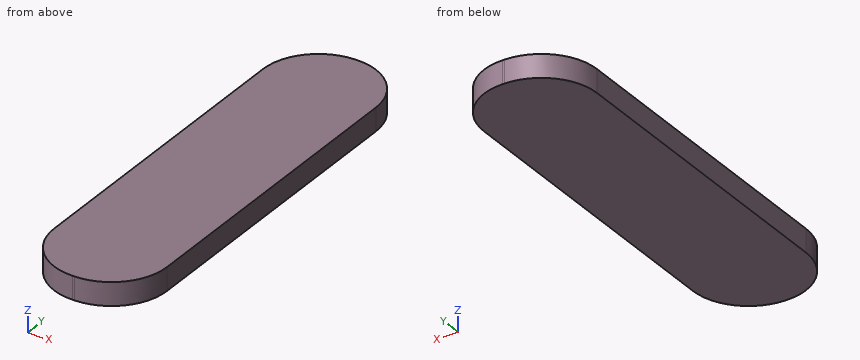
```python
from build123d import *

# Parameters (mm, degrees)
SKETCH1_W           = 12.2
SKETCH1_H           = 45.8
BOSS_EXTRUDE1_DEPTH = 2.5
FILLET1_R           = 6


with BuildPart() as part:
    # Sketch1 → Boss-Extrude1 (new body)
    with BuildSketch(Plane.XY.offset(10)):
        with Locations((-182.131179691, 159.988166791)):
            Rectangle(SKETCH1_W, SKETCH1_H)
    extrude(amount=BOSS_EXTRUDE1_DEPTH)

    # Fillet1
    fillet1_edges = [part.edges().sort_by_distance(p)[0] for p in [
        (-188.231179691, 182.888166791, 11.25),
        (-176.031179691, 182.888166791, 11.25),
        (-176.031179691, 137.088166791, 11.25),
        (-188.231179691, 137.088166791, 11.25),
    ]]
    fillet(fillet1_edges, radius=FILLET1_R)


solid = part.part
```
Geometry: final body of the model. Coordinates: model frame, mm. Coordinates: 2 decimals unless noted, no trailing zeros. Order: outer loops, then holes, each group sorted by start corner. A loop starts at its lowest first (then second) coordinate and runs counter-clockwise, first axis right, second up. Notation, with made-up numbers: M 74,58.5 L 119,58.5 A32 ccw 119,95.5 Z; hole C 84,30.5 d7. An arc over 180 degrees is marked long. Answer as CSV lines item,"result".
Q1. Section C-C on y = 142. Return the cut outline in (x, z), and give its area (3 significant figures).
Answers:
outline,"M -188.13,10 L -176.13,10 L -176.13,12.5 L -188.13,12.5 Z"
area,"30.0 mm^2"
Q2. Section A-A on z = 11.5. Return the cut outline in (x, y).
Answers:
outline,"M -188.23,143.09 A6 ccw -182.23,137.09 L -182.03,137.09 A6 ccw -176.03,143.09 L -176.03,176.89 A6 ccw -182.03,182.89 L -182.23,182.89 A6 ccw -188.23,176.89 Z"
Q3. Line query: probe 1 along Y at (x, z) = (-179.75, 11.15); probe 2 along Y at (x, z) = (-181.5, 11.65); probe 3 along X at (y, z) = (180.5, 11.8). Output: solid intervals per line, ascending. Write a range as [from, to].
Answers:
probe 1,"y = [137.54, 182.44]"
probe 2,"y = [137.11, 182.86]"
probe 3,"x = [-187.02, -177.24]"
Q4. Section B-B on x = -178.75. Return the cut outline in (y, z).
Answers:
outline,"M 138.06,10 L 181.91,10 L 181.91,12.5 L 138.06,12.5 Z"
